Build history of the part. All positions in model axes, mm. A direction names the side the tool comes from. Round coordinates to 2 decimals unless told otherwise and drop trailing zeros. Loops run counter-clockwise (first coordinate to the right, second up) from the corner with the lowest first, then second, coordinate; pieces in that order, holes last.
from build123d import *

# Parameters (mm, degrees)
F3_D     = 2.2606
F3_DEPTH = 6.351


with BuildPart() as f1:
    # F0 (on Front) → F1 (revolve)
    with BuildSketch(Plane.XZ):
        Polygon((-7.6835, 1.27), (-7.6835, 0), (-3.2385, 0), (-3.2385, -6.35), (0, -6.35), (0, 19.05), align=None)
    revolve(axis=Axis((0, 0, 6.35), (0, 0, 1)))

    # F3 (through all, one way)
    with BuildSketch(Plane.XY):
        with Locations((0, 0)):
            Circle(F3_D / 2)
    extrude(amount=-F3_DEPTH, mode=Mode.SUBTRACT)


solid = f1.part
(1) Slice it at B-B on z = 16. List the corners of the cut face in (x, y), plus the area to 3 significant figures.
Responses:
outline: circle Ø2.64 at (0, 0)
area: 5.46 mm2
(2) Pin check, flat tips, straight feed: P1, Ø6, axis at x = -5.5, y = -5, coming from the -Z side; P2, Ø5, axis at y = -2.5, z = 10.5, coming from the +X side; P3, Ø1, axis at y = 0, z = 16, coming from the +X side. Stop position of each tip, or through.
Responses:
P1: stops at z = 0
P2: stops at x = 4.46
P3: stops at x = 1.53
(3) Slice it at C-C on z = 7.5. List the corners of the cut face in (x, y), plus the area to 3 significant figures.
Responses:
outline: circle Ø9.98 at (0, 0)
area: 78.3 mm2
(4) Slice it at A-A on z = -3. List the corners of the cut face in (x, y).
Responses:
outline: circle Ø6.48 at (0, 0); hole circle Ø2.26 at (0, 0)
(5) Pull direction X, two halves, no side cores. Call faces 3 (the face through (-0.245, -1.103, -3.131)), 4 (the face through (-7.33, -2.31, 0.63)), 5 (the face through (-2, 3, 0)): +X half, -X half, draft (parallel to the pull), parting line (faces both ways), or undercut.
Responses:
face 3: undercut
face 4: parting line
face 5: draft
(6) Which spindle directions (+Z, -Z, +X, -X, +Y, -Y) get a long thin tool onto all of the face, cutting with end or side? Do faces 1 (the face through (-1.4, 2.7, 12.01)), 2 (the face through (0, 0, 0)). Say none if no direction does.
Responses:
face 1: +Z
face 2: -Z
(7) Probe line 1 (Y direction, x = 0, z = -3.25); line 2 (Y direction, x = -0.5, z = -3); line 3 (Z direction, x = 6, y = 3.75). List the from-to ranges inside material, lowest first.
Responses:
line 1: y = -3.24 to -1.13, 1.13 to 3.24
line 2: y = -3.2 to -1.01, 1.01 to 3.2
line 3: z = 0 to 2.68
